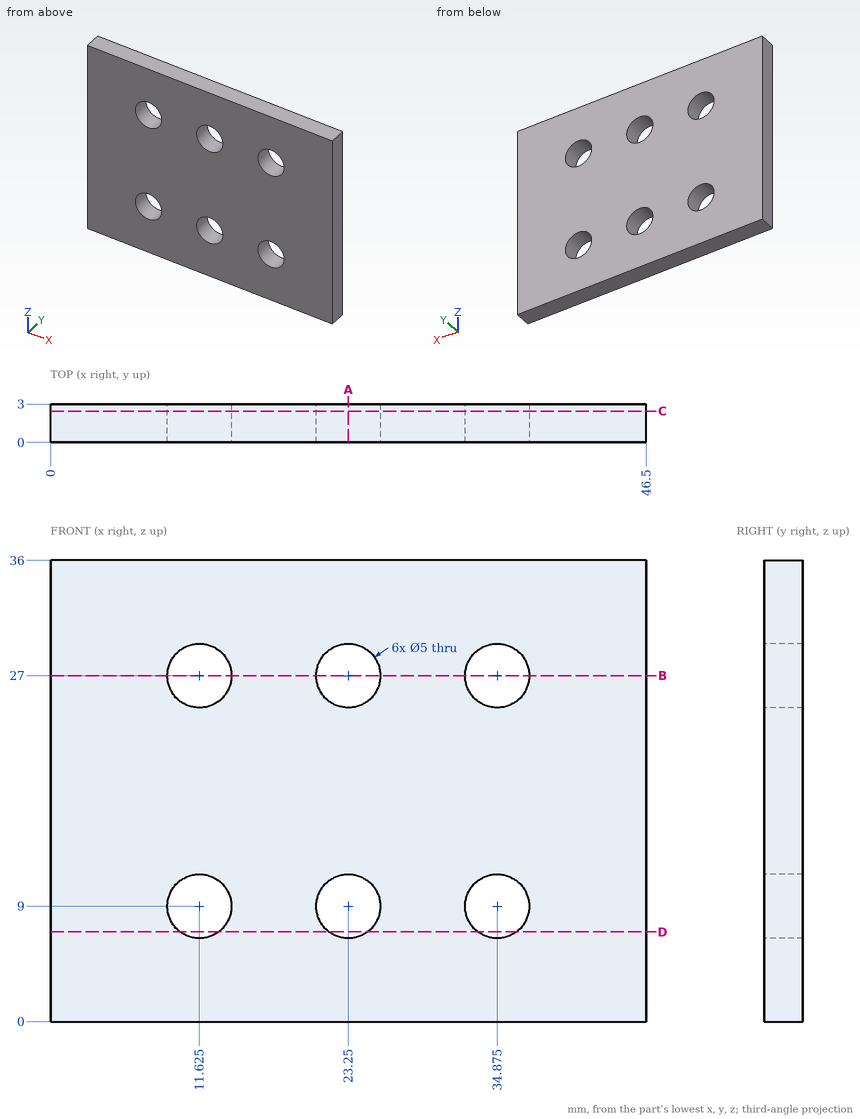
Verification items for this drawing (mm, ordinates from the low corner). Round coordinates to 2 decimals unless told otherwise and drop trailing zeros. Write each loop counter-clockwise with the first axis right and the second up, starting at its lowest first coordinate (ties: lowest second). Pieces come first, ordered by that corner, then holes. Notation, with made-up numbers: (-33, -24.75) - (13, -24.75) arc R16 ccw to (13, 4.25) - close; hole circle Ø7 at (0.5, 21.5). An arc over 180 degrees is marked (long way). One line per item, written item: value.
1. Cross-section at C-C on y = 2.45. Record the boundary of the cut face in (x, z) (3 decimals).
The answers:
outline: (0, 0) - (46.5, 0) - (46.5, 36) - (0, 36) - close; hole circle Ø5 at (11.625, 9); hole circle Ø5 at (11.625, 27); hole circle Ø5 at (23.25, 9); hole circle Ø5 at (23.25, 27); hole circle Ø5 at (34.875, 9); hole circle Ø5 at (34.875, 27)
2. Cross-section at A-A on x = 23.25. Record the boundary of the cut face in (y, z).
The answers:
outline: (0, 0) - (3, 0) - (3, 6.5) - (0, 6.5) - close; (0, 11.5) - (3, 11.5) - (3, 24.5) - (0, 24.5) - close; (0, 29.5) - (3, 29.5) - (3, 36) - (0, 36) - close
3. Depth check by flat-ended pin: pin 1 Ø4.5 at (x, z) = (23.25, 27) entering from +Y. Enter the tip coordinate at first touch or a pass-through.
The answers:
pin 1: passes through
4. Scan lines: L1, parallel to Z at x = 23.25, y = 2.3; L2, parallel to X at y = 2.35, z = 25.5 (3 decimals). Record each from-to range of solid material in increasing order.
The answers:
L1: z = 0 to 6.5, 11.5 to 24.5, 29.5 to 36
L2: x = 0 to 9.625, 13.625 to 21.25, 25.25 to 32.875, 36.875 to 46.5
5. Cross-section at B-B on z = 27. Record the boundary of the cut face in (x, y) (3 decimals).
The answers:
outline: (0, 0) - (9.125, 0) - (9.125, 3) - (0, 3) - close; (14.125, 0) - (20.75, 0) - (20.75, 3) - (14.125, 3) - close; (25.75, 0) - (32.375, 0) - (32.375, 3) - (25.75, 3) - close; (37.375, 0) - (46.5, 0) - (46.5, 3) - (37.375, 3) - close
6. Cross-section at D-D on z = 7. Record the boundary of the cut face in (x, y) (3 decimals).
The answers:
outline: (0, 0) - (10.125, 0) - (10.125, 3) - (0, 3) - close; (13.125, 0) - (21.75, 0) - (21.75, 3) - (13.125, 3) - close; (24.75, 0) - (33.375, 0) - (33.375, 3) - (24.75, 3) - close; (36.375, 0) - (46.5, 0) - (46.5, 3) - (36.375, 3) - close
